```python
from build123d import *

# Parameters (mm, degrees)
F0_W     = 38.1
F0_H     = 506.73
F1_DEPTH = 274.6375
F2_T     = -2.778125
F3_R     = 2.5796875
F3_W     = 11.1125
F3_H     = 11.1125
F4_DEPTH = 506.731
F5_R     = 3.175
F6_DEPTH = 549.276


# Not quite as in the source:
# - a feature names something its author has since deleted; it is built from what else it names


with BuildPart() as f1:
    # F0 (on Top) → F1 (new body, symmetric)
    with BuildSketch(Plane.XY):
        with Locations((19.05, 253.365)):
            Rectangle(F0_W, F0_H)
    extrude(amount=F1_DEPTH, both=True)

    # F2
    f2_openings = [f1.faces().sort_by_distance(p)[0] for p in [
        (38.1, 253.365, 0),
    ]]
    offset(amount=F2_T, openings=f2_openings)

    # F3 (on face) → F4 (cut, through all)
    with BuildSketch(Plane(origin=(0, 506.73, 0), x_dir=(-1, 0, 0), z_dir=(0, 1, 0))):
        with Locations((-19.05, 252.4125)):
            Circle(F3_R)
        with Locations((-19.05, 0)):
            Circle(F3_R)
        with Locations((-19.05, -252.4125)):
            Circle(F3_R)
        with Locations((-25.4, 219.075)):
            Rectangle(F3_W, F3_H)
        with Locations((-25.4, -219.075)):
            Rectangle(F3_W, F3_H)
    extrude(amount=-F4_DEPTH, mode=Mode.SUBTRACT)

    # F5 (on face) → F6 (cut, through all)
    with BuildSketch(Plane.XY.offset(274.6375)):
        with Locations((19.05, 481.33)):
            Circle(F5_R)
        with Locations((19.05, 253.365)):
            Circle(F5_R)
        with Locations((19.05, 25.4)):
            Circle(F5_R)
    extrude(amount=-F6_DEPTH, mode=Mode.SUBTRACT)


solid = f1.part
```
Work out the finished part from the listing and answer in its coordinate system (mm). A direction names the side the tool comes from. Give positions to 0.01 mm unless a question says otherwise; leave off trailing zeros. Write each loop counter-clockwise with the first axis right and the second up, starting at its lowest first coordinate (ties: lowest second). Pieces come first, ordered by that corner, then holes.
(1) Which of the six approach directions +Z, -Z, +X, -X, +Y, -Y give full straight-line access (tool end or side, diameter ignored) to faces 1 (the flat face through (20, 257, -271.859)), 2 (the flat face through (19, 257, 274.638))?
Final values:
face 1: +X
face 2: +Z, +X, -X, +Y, -Y
(2) The part is cut by section A-A on y = 307.5. Write down the section's boundary in (x, z).
Final values:
outline: (0, -274.64) - (38.1, -274.64) - (38.1, -271.86) - (2.78, -271.86) - (2.78, 271.86) - (38.1, 271.86) - (38.1, 274.64) - (0, 274.64) - close
(3) Flat-ended cylindrical pins translate along their axes: pin 1 Ø4 at (x, y) = (19.05, 253.365) entering from +Z; pin 2 Ø6 at (y, z) = (338, -195) entering from +X. Find the tip coordinate at first contact, or state that the pin passes through.
Final values:
pin 1: passes through
pin 2: stops at x = 2.78
(4) The part is cut by section B-B on z = 18. Write down the section's boundary in (x, y), plus the area to 3 significant figures.
Final values:
outline: (0, 0) - (38.1, 0) - (38.1, 2.78) - (2.78, 2.78) - (2.78, 503.95) - (38.1, 503.95) - (38.1, 506.73) - (0, 506.73) - close
area: 1,600 mm2
(5) Straight lines are drawn through the part: line 1 (Z direction, x = 19.05, y = 505.4); line 2 (Y direction, x = 19.05, z = 273.2) (3 decimals); line 3 (Y direction, x = 6, z = 148). For each, find the intervals that lie inside material, in ascending order.
Final values:
line 1: z = -274.64 to -254.99, -249.83 to -2.58, 2.58 to 249.83, 254.99 to 274.64
line 2: y = 0 to 22.225, 28.575 to 250.19, 256.54 to 478.155, 484.505 to 506.73
line 3: y = 0 to 2.78, 503.95 to 506.73
(6) The mould has two halves that part along Y. Classify faces 3 (the flat face through (19, 0, 4)), 4 (the flat face through (19, 506.73, 4)), 5 (the flat face through (20, 503.952, 4)), 6 (the flat face through (0, 250, 4)): pulls with the +Y half, pulls with the -Y half, needs draft (parallel to the pull), parting line crosses it, or undercut.
Final values:
face 3: pulls with the -Y half
face 4: pulls with the +Y half
face 5: undercut
face 6: needs draft
